```python
from build123d import *

# Parameters (mm, degrees)
F1_DEPTH = 20


with BuildPart() as f1:
    # F0 (on Front) → F1 (new body)
    with BuildSketch(Plane.XZ):
        with BuildLine():
            Line((0, 10), (0, 0))
            Line((0, 0), (150, 0))
            Line((150, 0), (150, 300))
            ThreePointArc((150, 300), (113.168588, 138.987578), (10, 10))
            Line((10, 10), (0, 10))
        make_face()
        with BuildLine():
            Line((150, 300), (150, 0))
            ThreePointArc((150, 0), (186.831412, 161.012422), (290, 290))
            Line((290, 290), (300, 290))
            Line((300, 290), (300, 300))
            Line((300, 300), (150, 300))
        make_face()
    extrude(amount=F1_DEPTH)


solid = f1.part
```
The model under review builds one solid part; all positions refer to its coordinate system, in mm. A direction names the side the tool comes from. Coordinates: 2 decimals unless noted, no trailing zeros. Write each loop counter-clockwise with the first axis right and the second up, starting at its lowest first coordinate (ties: lowest second). Pieces come first, ordered by that corner, then holes. Notation, with made-up numbers: (69, 30) -> (89, 30) arc R29 cw to (89, 65) -> close; hole circle Ø7 at (86.5, 77). An arc over 180 degrees is marked (long way). One line per item, written item: value. Start each with the question number.
Q1. The part is to be moulded in two halves that separate along Y. For faces 1 (the face through (114.176, -9.86, 141.091)), 2 (the face through (149, -20, 140)), 3 (the face through (149, 0, 140)), say which applies: +Y half, -Y half, draft (parallel to the pull), parting line (faces both ways), or undercut.
Q2. Add section B-B, the plane z = 103. Give the boundary of the cut face in (x, y), then the cut area to 3 significant figures.
Q3. For faces 4 (the face through (295, -10, 290)), 5 (the face through (74, -10, 0)), 6 (the face through (5, -10, 10)), list the 3-axis set-ups (+Z, -Z, +X, -X, +Y, -Y) from which the entire face can be reached by the end or side of a thin tool; tool diameter is ignored.
Q4. Add section A-A, the plane y = -15. Give the boundary of the cut face in (x, z), then the cut area to 3 significant figures.
Q5. Clearance check with flat-ended pins moving along their axes: P1, Ø3, axis at x = 3.5, y = -12.5, coming from the +Z side; P2, Ø3, axis at x = 297, y = -8, coming from the -Z side; P3, Ø2, axis at x = 127, z = 86.5, coming from the +Y side; P4, Ø5, axis at y = -13, z = 61.5, coming from the -X side. State where each tip first meets the part, or that it passes through.
Q6. Add section C-C, the plane x = 85.5. Give the boundary of the cut face in (y, z), then the cut area to 3 significant figures.
Q7. To check wall thickness, follow probe 1 along X at (y, z) = (-8, 93.5); probe 2 along X at (y, z) = (-18.5, 65); probe 3 along Z at (x, y) = (44, -19). State the ranges of each line that lie inside material, in increasing order.
Response:
1. face 1: draft
1. face 2: -Y half
1. face 3: +Y half
2. outline: (93.26, -20) -> (164.61, -20) -> (164.61, 0) -> (93.26, 0) -> close
2. area: 1,430 mm²
3. face 4: -Z, +X, +Y, -Y
3. face 5: -Z, +X, -X, +Y, -Y
3. face 6: +Z, -X, +Y, -Y
4. outline: (0, 0) -> (150, 0) arc R370.36 cw to (290, 290) -> (300, 290) -> (300, 300) -> (150, 300) arc R370.36 cw to (10, 10) -> (0, 10) -> close
4. area: 27,600 mm²
5. P1: z = 10
5. P2: z = 290
5. P3: y = 0
5. P4: x = 60.86
6. outline: (-20, 0) -> (0, 0) -> (0, 91.16) -> (-20, 91.16) -> close
6. area: 1,820 mm²
7. probe 1: 87.09 to 162
7. probe 2: 65.89 to 155.75
7. probe 3: 0 to 40.62
